Part model, mm, in its own coordinate system. A direction names the side the tool comes from. Give positions to 0.01 mm unless a question says otherwise; leave off trailing zeros. Write each loop counter-clockwise with the first axis right and the second up, starting at its lowest first coordinate (ties: lowest second). Pieces come first, ordered by that corner, then holes.
from build123d import *

# Parameters (mm, degrees)
SKETCH1_R           = 16.2
BOSS_EXTRUDE1_DEPTH = 7.1
SKETCH6_R           = 13.2
SKETCH6_R_2         = 4.5
CUT_EXTRUDE2_DEPTH  = 6.1
FILLET2_R           = 0.5
FILLET3_R           = 0.5
FILLET4_R           = 0.5
FILLET5_R           = 0.5
SKETCH7_R           = 2.5
CUT_EXTRUDE3_DEPTH  = 27.954035009


with BuildPart() as part:
    # Sketch1 → Boss-Extrude1 (new, symmetric)
    with BuildSketch(Plane(origin=(0, 0, 0), x_dir=(0, 0, -1), z_dir=(1, 0, 0))):
        Circle(SKETCH1_R)
    extrude(amount=BOSS_EXTRUDE1_DEPTH, both=True)

    # Sketch6 → Cut-Extrude2 (cut)
    with BuildSketch(Plane.ZY.offset(7.1)):
        Circle(SKETCH6_R)
        Circle(SKETCH6_R_2, mode=Mode.SUBTRACT)
    cut_extrude2 = extrude(amount=-CUT_EXTRUDE2_DEPTH, mode=Mode.SUBTRACT)

    # Mirror1: Cut-Extrude2 across plane
    add(cut_extrude2.mirror(Plane(origin=(0, 0, 0), x_dir=(0, 0, 1), z_dir=(1, 0, 0))), mode=Mode.SUBTRACT)

    # Fillet2
    fillet2_edges = [part.edges().sort_by_distance(p)[0] for p in [
        (-7.1, 0, 16.2),
    ]]
    fillet(fillet2_edges, radius=FILLET2_R)

    # Fillet3
    fillet3_edges = [part.edges().sort_by_distance(p)[0] for p in [
        (-7.1, 0, -13.2),
    ]]
    fillet(fillet3_edges, radius=FILLET3_R)

    # Fillet4
    fillet4_edges = [part.edges().sort_by_distance(p)[0] for p in [
        (7.1, 0, -13.2),
    ]]
    fillet(fillet4_edges, radius=FILLET4_R)

    # Fillet5
    fillet5_edges = [part.edges().sort_by_distance(p)[0] for p in [
        (7.1, 0, 16.2),
    ]]
    fillet(fillet5_edges, radius=FILLET5_R)

    # Sketch7 → Cut-Extrude3 (cut, through all)
    with BuildSketch(Plane.ZY.offset(7.1)):
        Circle(SKETCH7_R)
    extrude(amount=-CUT_EXTRUDE3_DEPTH, mode=Mode.SUBTRACT)


solid = part.part
1) 3-axis set-ups, long thin cutter, end or side, ignore diameter. For faces 5 (the flat face through (1, 0, 6)), 6 (the cylindrical face through (-3.84, 8.92, -9.73)), 7 (the flat face through (-7.1, 13, 5)): which of +Z, -Z, +X, -X, +Y, -Y reach the whole face in a straight line?
Check result:
face 5: +X
face 6: -X
face 7: +Z, -Z, -X, +Y, -Y
2) Flat gauge pins, fed straight in: P1, Ø6, axis at x = 1.5, z = 5, coming from the +Y side; P2, Ø6, axis at y = 7, z = -2, coming from the -X side; P3, Ø3, axis at x = 2, y = 10.5, coming from the +Z side; P4, Ø4, axis at x = 0, z = -2.5, coming from the -Y side. Where does each tip first touch, or does it go through?
Check result:
P1: stops at y = 16.08
P2: stops at x = -7.1
P3: stops at z = 13.47
P4: stops at y = -16.19
3) Mould opens along Y. For faces 1 (the flat face through (7.1, 13, 5)), 2 (the cylindrical face through (-0.1, -2.44, -0.54)), 3 (the cylindrical face through (0.092, -15.815, 3.512)), 4 (the cylindrical face through (3.84, 8.92, -9.73)) say: +Y half, -Y half, draft (parallel to the pull), parting line (faces both ways), or undercut.
Check result:
face 1: draft
face 2: undercut
face 3: parting line
face 4: undercut
4) Drill centre lines: L1, parallel to Y at x = 4.8, z = 0; L2, parallel to Z at x = 5.5, y = -3.5; L3, parallel to Y at x = 3.75, z = 1.5. Where is each one in solid material? Low to high.
Check result:
L1: y = -16.2 to -13.2, -4.5 to -2.5, 2.5 to 4.5, 13.2 to 16.2
L2: z = -15.82 to -12.73, -2.83 to 2.83, 12.73 to 15.82
L3: y = -16.13 to -13.11, -4.24 to -2, 2 to 4.24, 13.11 to 16.13
5) Saw through at C-C (x = -2.25). Write the cut outline in (y, z), and give its area (3 significant figures).
Check result:
outline: circle Ø32.4 at (0, 0); circle Ø9 at (0, 0); hole circle Ø26.4 at (0, 0); hole circle Ø5 at (0, 0)
area: 321 mm2
